CAD build for the part. Positions are in the model's coordinates, mm. A direction names the side the tool comes from. Give positions to 0.01 mm unless a question says otherwise; leave off trailing zeros. Loops run counter-clockwise (first coordinate to the right, second up) from the corner with the lowest first, then second, coordinate; pieces in that order, holes last.
Item 1: Probe probe 1 along Z at (x, y) = (16.35, 0) (3 decimals); probe 2 along X at (y, z) = (10.5, 3); probe 3 along Y at (x, z) = (0, -0.5). List the from-to ranges inside material, lowest first.
Item 2: Saw through at C-C on z = 2.25. Give the cut face in (x, y), plus the area to 3 significant figures.
Item 3: Which spindle directions (+Z, -Z, +X, -X, +Y, -Y) get a long thin tool onto all of the face, cutting with end or side? Do faces 1 (the flat face through (-15, 7, 3.175)), 2 (the cylindrical face through (16.604, 1.525, -0.632)). Say none if no direction does.
Item 4: Saw through at A-A on y = 0. Give the cut face in (x, z) (3 decimals), plus the area to 3 significant figures.
Item 5: Saw through at B-B on x = 0. Give the cut face in (y, z) (3 decimals).
Item 6: Drop flat-ended pins along their axis: P1, Ø2, axis at y = 9.5, z = 2.5, coming from the -X side; P2, Ø3, axis at y = -3.5, z = 0.5, coming from the -X side; P3, Ø1, axis at y = 2, z = 2, coming from the +X side; P4, Ø1, axis at x = -2, y = -13.5, coming from the -Z side. Give the stop position or say it passes through.
Item 7: Mould opens along Z. For faces 3 (the cylindrical face through (-16.584, -0.215, 1.637)), 4 (the flat face through (-15, 7, -3.175)), 5 (the flat face through (17.272, 0, 0)), 6 (the cylindrical face through (-13.716, -11.642, -0.608)) say: released by +Z, released by -Z, zero draft, split by the parting line, or undercut.
Item 8: Saw through at D-D on y = 4. Give the cut face in (x, z) (3 decimals).
from build123d import *

# Parameters (mm, degrees)
F1_R     = 17.78
F2_DEPTH = 3.175
F3_R     = 1.651
F4_DEPTH = 17.272
F5_R     = 1.5875
F6_DEPTH = 19.431
F7_R     = 16.002
F8_DEPTH = 6.3510001
F9_R     = 1.27


with BuildPart() as f2:
    # F1 (on Top) → F2 (new body, symmetric)
    with BuildSketch(Plane.XY):
        Circle(F1_R)
    extrude(amount=F2_DEPTH, both=True)

    # F3 (on Right) → F4 (cut, symmetric)
    with BuildSketch(Plane.YZ):
        Circle(F3_R)
    extrude(amount=F4_DEPTH, both=True, mode=Mode.SUBTRACT)

    # F5 (on face) → F6 (join, symmetric)
    with BuildSketch(Plane(origin=(0, 0, 0), x_dir=(-0.7071067812, 0.7071067812, 0), z_dir=(0.7071067812, 0.7071067812, 0))):
        Circle(F5_R)
    extrude(amount=F6_DEPTH, both=True)

    # F7 (on face) → F8 (cut, through all)
    with BuildSketch(Plane.XY.offset(3.175)):
        Circle(F7_R)
    extrude(amount=-F8_DEPTH, mode=Mode.SUBTRACT)

    # F9
    f9_edges = [f2.edges().sort_by_distance(p)[0] for p in [
        (14.862324, 12.61726, 0),
        (-12.61726, -14.862324, 0),
    ]]
    fillet(f9_edges, radius=F9_R)


solid = f2.part
Results below:
1. probe 1: z = -3.175 to -1.651, 1.651 to 3.175
1. probe 2: x = -14.35 to -12.08, 12.08 to 14.35
1. probe 3: y = -17.78 to -16, 16 to 17.78
2. outline: circle Ø35.56 at (0, 0); hole circle Ø32 at (0, 0)
2. area: 189 mm2
3. face 1: +Z, +X, -X, +Y, -Y
3. face 2: none
4. outline: (-17.78, -3.175) - (-16.002, -3.175) - (-16.002, -1.651) - (-17.272, -1.651) - (-17.272, 1.651) - (-16.002, 1.651) - (-16.002, 3.175) - (-17.78, 3.175) - close; (16.002, -3.175) - (17.78, -3.175) - (17.78, 3.175) - (16.002, 3.175) - (16.002, 1.651) - (17.272, 1.651) - (17.272, -1.651) - (16.002, -1.651) - close
4. area: 14.2 mm2
5. outline: (-17.78, -3.175) - (-16.002, -3.175) - (-16.002, 3.175) - (-17.78, 3.175) - close; (16.002, -3.175) - (17.78, -3.175) - (17.78, 3.175) - (16.002, 3.175) - close
6. P1: stops at x = -15.62
6. P2: stops at x = -17.67
6. P3: stops at x = 17.72
6. P4: passes through
7. face 3: undercut
7. face 4: released by -Z
7. face 5: undercut
7. face 6: split by the parting line
8. outline: (-17.324, -3.175) - (-15.494, -3.175) - (-15.494, 3.175) - (-17.324, 3.175) - close; (15.494, -3.175) - (17.324, -3.175) - (17.324, 3.175) - (15.494, 3.175) - close
